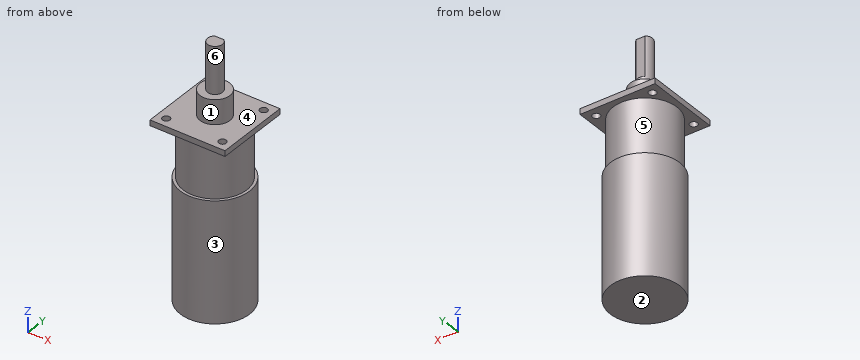
Autodesk Inventor part; units mm, degrees
ref_plane "YZ Plane" through (0, 0, 0) normal (1, 0, 0) x (0, 1, 0)
ref_plane "XZ Plane" through (0, 0, 0) normal (0, 1, 0) x (-1, 0, 0)
ref_plane "XY Plane" through (0, 0, 0) normal (0, 0, 1) x (1, 0, 0)
sketch "Sketch1" plane through (0, 0, 0) normal (0, 0, 1) x (1, 0, 0)
  line L0 (0, 0) -> (40, 0)
  line L1 (40, 0) -> (40, 40)
  line L2 (40, 40) -> (0, 40)
  line L3 (0, 40) -> (0, 0)
  dimension "d0" = 40
  dimension "d1" = 40
extrude "Extrusion1" add sketch "Sketch1" along normal blind 3
sketch "Sketch2" plane through (0, 0, 3) normal (0, 0, 1) x (1, 0, 0)
  line L0 (40, 0) -> (0, 0)
  line L1 (40, 40) -> (40, 0)
  line L2 (35, 5) -> (5, 5)
  line L3 (5, 5) -> (5, 35)
  line L4 (5, 35) -> (35, 35)
  line L5 (35, 35) -> (35, 5)
  circle A0 centre (20, 20) radius 8
  dimension "d4" = 30
  dimension "d5" = 30
  dimension "d6" = 5
  dimension "d7" = 5
  dimension "d8" = 16
extrude "Extrusion2" add sketch "Sketch2" along normal blind 13 contours A0
sketch "Sketch3" plane through (0, 0, 3) normal (0, 0, 1) x (1, 0, 0)
  line L0 (40, 0) -> (0, 0)
  line L1 (40, 40) -> (40, 0)
  line L2 (5, 5) -> (35, 5)
  line L3 (35, 5) -> (35, 35)
  line L4 (35, 35) -> (5, 35)
  line L5 (5, 35) -> (5, 5)
  dimension "d11" = 30
  dimension "d12" = 30
  dimension "d13" = 5
  dimension "d14" = 5
hole "Hole1" at (5, 5, 3) at (35, 5, 3) at (35, 35, 3) at (5, 35, 3) direction (0, 0, -1) diameter 4 end through all
sketch "Sketch4" plane through (20, 20, 16) normal (0, 0, 1) x (1, 0, 0)
  circle A0 centre (0, 0) radius 8
  circle A1 centre (0, 0) radius 4
  point P0 (-20, -20)
  dimension "d22" = 8
extrude "Extrusion3" add sketch "Sketch4" along normal blind 25 contours A1
sketch "Sketch5" plane through (20, 20, 41) normal (0, 0, 1) x (1, 0, 0)
  circle A0 centre (0, 0) radius 4
  line L0 (-4, 0) -> (4, 0)
  line L1 (4, 0) -> (4, 4)
  line L2 (4, 4) -> (-4, 4)
  line L3 (-4, 4) -> (-4, 0)
  line L4 (-4, 4) -> (4, 4)
  line L5 (4, 4) -> (4, 3.2)
  line L6 (4, 3.2) -> (-4, 3.2)
  line L7 (-4, 3.2) -> (-4, 4)
  point P0 (-20, -20)
  dimension "d25" = 0.8
extrude "Extrusion4" cut sketch "Sketch5" against normal blind 21 contours L6 L3 L2 A0 | A0 L6 | A0 L2 L1 L6
sketch "Sketch6" plane through (0, 0, 0) normal (0, 0, -1) x (-1, 0, 0)
  circle A0 centre (-20, 20) radius 17
  dimension "d28" = 34
extrude "Extrusion5" add sketch "Sketch6" along normal blind 29.5
sketch "Sketch7" plane through (20, 20, -29.5) normal (0, 0, -1) x (-1, 0, 0)
  circle A0 centre (0, 0) radius 17
  circle A1 centre (0, 0) radius 18.5
  point P0 (20, -20)
  dimension "d31" = 37
extrude "Extrusion6" add sketch "Sketch7" along normal blind 64 contours A0 | A1
properties part number "mr85vel 2 etapas" material "UHMW, White"
Here's how the part is built. I have some questions about the finished solid (model axes, mm). Face numbers are marked on the shaded views. A direction names the side the tool comes from. Give positions to 0.01 mm unless a question says otherwise; leave off trailing zeros. Loops run counter-clockwise (first coordinate to the right, second up) from the corner with the lowest first, then second, coordinate; pieces in that order, holes last. Notation, with made-up numbers: M -21,-37 L -13,-37 A31 cw -13,0 Z; hole C -22.5,-2 d1. An arc over 180 degrees is marked long. Use one line per item in the form item = value. Start each with the question number.
Q1. If we section it at C-C (y = 20): Write out the boundary of the cut face in (x, z), then the cut area to 3 significant figures.
Q2. If we section it at A-A (y = 35): Write out the boundary of the cut face in (x, z), then the cut area to 3 significant figures.
Q3. I need wall thicknesses on line 1 along Y through (x, z) = (35, 1.5); line 2 along Z through (x, y) = (13, 34). Which ranges of each line are inside material? Lowest first, please.
Q4. Which directions (+Z, -Z, +X, -X, +Y, -Y) give clear straight access to the entire face, cutting with the end or side of a thin tool? Please do the marked faces 1, 2 and 3.
Q5. Thinking about a two-plate mould opening in Z: for the marked faces 4, 5 and 6, which applies, +Z half, -Z half, draft (parallel to the pull), parting line (faces both ways), or undercut?
Q6. Will these pins go through, and if not, where does the flat tip stop? pin 1 Ø13 at (x, y) = (21.5, 16) entering from +Z; pin 2 Ø4.5 at (x, y) = (5, 35) entering from -Z; pin 3 Ø4 at (x, z) = (5.5, -27) entering from +Y; pin 4 Ø12 at (y, z) = (35.5, -76.5) entering from +X.
Q7. If we section it at D-D (x = 19.5): Write out the boundary of the cut face in (y, z).
Taken from the geometry:
q1.outline = M 0,0 L 3,0 L 3,-29.5 L 1.5,-29.5 L 1.5,-93.5 L 38.5,-93.5 L 38.5,-29.5 L 37,-29.5 L 37,0 L 40,0 L 40,3 L 28,3 L 28,16 L 24,16 L 24,41 L 16,41 L 16,16 L 12,16 L 12,3 L 0,3 Z
q1.area = 3,900 mm^2
q2.outline = M 0,0 L 3,0 L 3,3 L 0,3 Z; M 7,0 L 12,0 L 12,-29.5 L 9.17,-29.5 L 9.17,-93.5 L 30.83,-93.5 L 30.83,-29.5 L 28,-29.5 L 28,0 L 33,0 L 33,3 L 7,3 Z; M 37,0 L 40,0 L 40,3 L 37,3 Z
q2.area = 1,950 mm^2
q3.line_1 = 0 to 3, 7 to 33, 37 to 40
q3.line_2 = -93.5 to 3
q4.face_1 = +Z
q4.face_2 = -Z, +X, -X, +Y, -Y
q4.face_3 = -Z
q5.face_4 = +Z half
q5.face_5 = undercut
q5.face_6 = draft
q6.pin_1 = 41
q6.pin_2 = 0
q6.pin_3 = 31.52
q6.pin_4 = 35.87
q7.outline = M 0,0 L 3.01,0 L 3.01,-29.5 L 1.51,-29.5 L 1.51,-93.5 L 38.49,-93.5 L 38.49,-29.5 L 36.99,-29.5 L 36.99,0 L 40,0 L 40,3 L 27.98,3 L 27.98,16 L 23.97,16 L 23.97,20 L 23.2,20 L 23.2,41 L 16.03,41 L 16.03,16 L 12.02,16 L 12.02,3 L 0,3 Z
